Answer from the drawing. Dimensions are ordinates in mm from the lowest x, y and z of the part. Give positions to 0.01 mm unless a question says otherwise; leave off trailing zeros. Order: outer loops, then holes, each group sorted by start corner. A loop starts at its lowest first (then second) coordinate and runs counter-clockwise, first axis right, second up. Notation, with made-up numbers: (-11, 19.25) -> (9, 19.25) arc R17 cw to (9, 51.25) -> close; hole circle Ø1 at (-12, -37.75). An arc over 180 degrees is marked (long way). Write item = value, one per line. Start each with the question number.
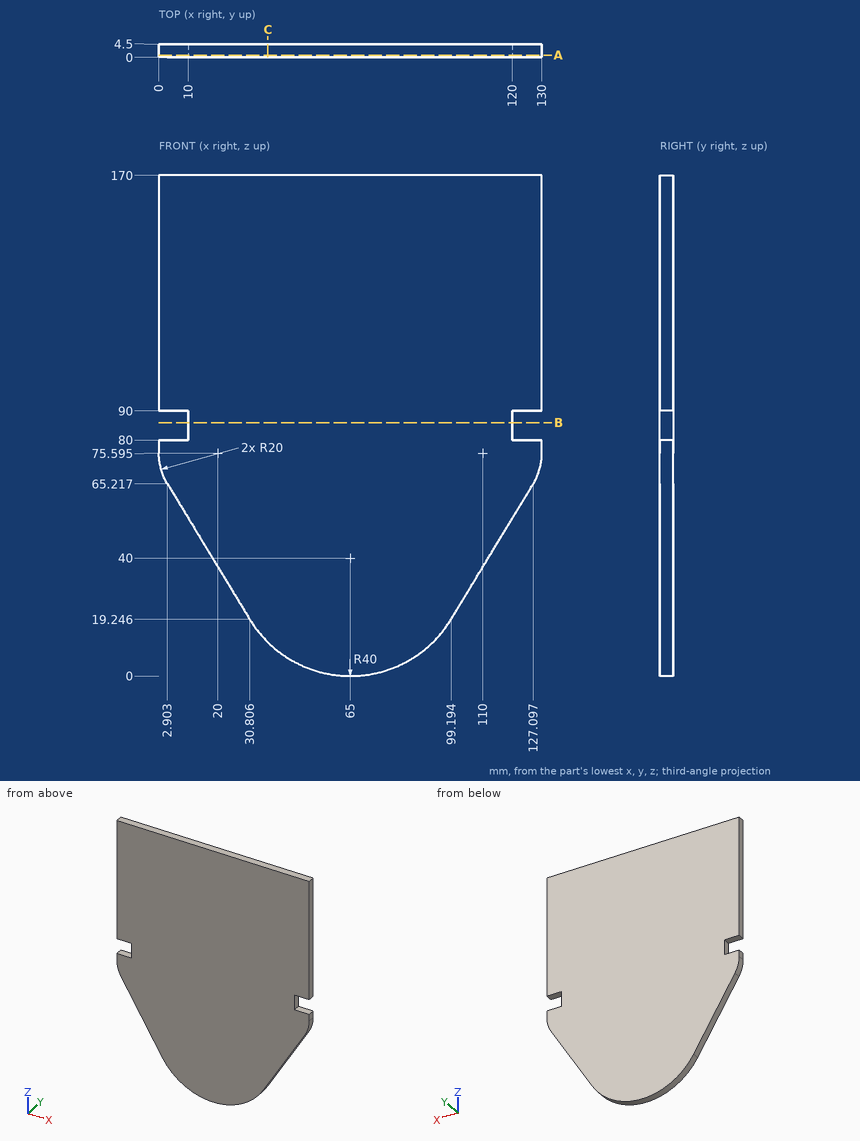
Item 1: Flat-ended cylindrical pins translate along their axes: pin 1 (1.3 mm diameter, centred on x = 124, y = 1.5, fed in from -Z) (1 decimal); pin 2 (1 mm diameter, centred on y = 1, z = 64.5, fed in from +X) (1 decimal); pin 3 (1 mm diameter, centred on x = 29.5, y = 1.5, fed in from -Z) (1 decimal). Find the tip coordinate at first contact, or state that the pin passes through.
Item 2: A cutting plane is placed at B-B, the plane z = 86. Write down the section's boundary in (x, y).
Item 3: A cutting plane is placed at C-C, the plane x = 37. Write down the section's boundary in (y, z) (1 decimal).
Item 4: A cutting plane is placed at A-A, the plane y = 0.7. Write down the section's boundary in (x, z) (1 decimal), plus the area to 3 significant figures.
Item 5: Consider L1, parallel to Z at x = 66, y = 0.65; L2, parallel to X at y = 3.55, z = 34; L3, parallel to Z at x = 71.5, y = 2.1. Determine where each line is inside the solid, lowest interval first. Write a range as from..to.
Check values:
q1.pin_1 = 59
q1.pin_2 = 127
q1.pin_3 = 20.6
q2.outline = (10, 0) -> (120, 0) -> (120, 4.5) -> (10, 4.5) -> close
q3.outline = (0, 11.4) -> (4.5, 11.4) -> (4.5, 170) -> (0, 170) -> close
q4.outline = (0, 75.6) arc R20 ccw to (2.9, 65.2) -> (30.8, 19.2) arc R40 ccw to (99.2, 19.2) -> (127.1, 65.2) arc R20 ccw to (130, 75.6) -> (130, 80) -> (120, 80) -> (120, 90) -> (130, 90) -> (130, 170) -> (0, 170) -> (0, 90) -> (10, 90) -> (10, 80) -> (0, 80) -> close
q4.area = 18,800 mm^2
q5.L1 = 0.01..170
q5.L2 = 21.85..108.15
q5.L3 = 0.53..170
